Input: part model. Units: mm. Frame: model coordinates. A direction names the side the tool comes from. Coordinates: 2 decimals unless noted, no trailing zeros. Order: outer loops, then holes, each group sorted by start corner. A loop starts at its lowest first (then second) coordinate and runs counter-clockwise, first axis right, second up. Notation, with made-up numbers: M 23,44 L 80,44 A13 cw 80,55 Z; hole C -12.5,10.5 d5. An arc over 180 degrees is marked long. Answer in a Markdown table with one row per item.
from build123d import *

# Parameters (mm, degrees)
SKETCH1_W           = 100
SKETCH1_H           = 100
SKETCH1_R           = 3.5
BOSS_EXTRUDE1_DEPTH = 5
CUT_EXTRUDE1_START  = -5
SKETCH6_R           = 5
CUT_EXTRUDE1_DEPTH  = 3
BOSS_EXTRUDE2_START = 40
SKETCH8_W           = 8
SKETCH8_H           = 58
BOSS_EXTRUDE2_DEPTH = 180
SKETCH9_W           = 180
SKETCH9_H           = 9
BOSS_EXTRUDE3_DEPTH = 230
SKETCH13_R          = 3.5
CUT_EXTRUDE3_DEPTH  = 9
SKETCH15_W          = 6
SKETCH15_H          = 100
BOSS_EXTRUDE6_DEPTH = 73
CUT_EXTRUDE4_REACH  = 309.259
SKETCH16_W          = 130
SKETCH16_H          = 25
FILLET1_R           = 40
FILLET2_R           = 10
SKETCH17_W          = 6
SKETCH17_H          = 20
BOSS_EXTRUDE7_DEPTH = 50
FILLET3_R           = 10
FILLET4_R           = 10
FILLET6_R           = 30
FILLET7_R           = 10
SKETCH18_W          = 10
SKETCH18_H          = 238
BOSS_EXTRUDE8_DEPTH = 20
FILLET8_R           = 10
FILLET9_R           = 10
FILLET10_R          = 5


# Some blends are built 0.0001 mm under size
with BuildPart() as part:
    # Sketch1 → Boss-Extrude1 (new body)
    with BuildSketch(Plane(origin=(0, 0, 0), x_dir=(1, 0, 0), z_dir=(0, 1, 0))):
        Rectangle(SKETCH1_W, SKETCH1_H)
        with Locations(Location((-37.5, 37.5, 0), (0, 0, 270))):
            Circle(SKETCH1_R, mode=Mode.SUBTRACT)
        with Locations(Location((37.5, 37.5, 0), (0, 0, 90))):
            Circle(SKETCH1_R, mode=Mode.SUBTRACT)
        with Locations(Location((37.5, -37.5, 0), (0, 0, 270))):
            Circle(SKETCH1_R, mode=Mode.SUBTRACT)
        with Locations(Location((-37.5, -37.5, 0), (0, 0, 90))):
            Circle(SKETCH1_R, mode=Mode.SUBTRACT)
    extrude(amount=BOSS_EXTRUDE1_DEPTH)

    # Sketch6 → Cut-Extrude1 (cut)
    with BuildSketch(Plane.XZ.offset(CUT_EXTRUDE1_START)):
        with Locations(Location((-37.5, 37.5, 0), (0, 0, 90))):
            Circle(SKETCH6_R)
        with Locations(Location((37.5, 37.5, 0), (0, 0, 90))):
            Circle(SKETCH6_R)
        with Locations(Location((37.5, -37.5, 0), (0, 0, 90))):
            Circle(SKETCH6_R)
        with Locations(Location((-37.5, -37.5, 0), (0, 0, 90))):
            Circle(SKETCH6_R)
    extrude(amount=CUT_EXTRUDE1_DEPTH, mode=Mode.SUBTRACT)

    # Sketch8 → Boss-Extrude2 (add)
    with BuildSketch(Plane.ZY.offset(50).offset(BOSS_EXTRUDE2_START)):
        with Locations((54, 29)):
            Rectangle(SKETCH8_W, SKETCH8_H)
    extrude(amount=-BOSS_EXTRUDE2_DEPTH)

    # Sketch9 → Boss-Extrude3 (add)
    with BuildSketch(Plane.XY.offset(58)):
        with Locations((0, 53.5)):
            Rectangle(SKETCH9_W, SKETCH9_H)
    extrude(amount=BOSS_EXTRUDE3_DEPTH)

    # Sketch13 → Cut-Extrude3 (cut)
    with BuildSketch(Plane(origin=(0, 58, 0), x_dir=(1, 0, 0), z_dir=(0, 1, 0))):
        with Locations(Location((-37.5, -190.5, 0), (0, 0, 270))):
            Circle(SKETCH13_R)
        with Locations(Location((37.5, -190.5, 0), (0, 0, 270))):
            Circle(SKETCH13_R)
        with Locations(Location((37.5, -265.5, 0), (0, 0, 270))):
            Circle(SKETCH13_R)
        with Locations(Location((-37.5, -265.5, 0), (0, 0, 270))):
            Circle(SKETCH13_R)
    extrude(amount=-CUT_EXTRUDE3_DEPTH, mode=Mode.SUBTRACT)

    # Sketch15 → Boss-Extrude6 (add)
    with BuildSketch(Plane(origin=(0, 5, 0), x_dir=(1, 0, 0), z_dir=(0, 1, 0))):
        with Locations((-47, 0)):
            Rectangle(SKETCH15_W, SKETCH15_H)
        with Locations((47, 0)):
            Rectangle(SKETCH15_W, SKETCH15_H)
    extrude(amount=BOSS_EXTRUDE6_DEPTH)

    # Sketch16 → Cut-Extrude4 (cut, up to next)
    with BuildSketch(Plane(origin=(0, 58, 0), x_dir=(1, 0, 0), z_dir=(0, 1, 0)), mode=Mode.PRIVATE) as cut_extrude4_sk1:
        with Locations((0, -130.5)):
            Rectangle(SKETCH16_W, SKETCH16_H)
    cut_extrude4_tool1 = extrude(cut_extrude4_sk1.sketch, amount=-CUT_EXTRUDE4_REACH, mode=Mode.PRIVATE) & part.part
    add(cut_extrude4_tool1.solids().sort_by_distance((0, 58, 130.5))[0], mode=Mode.SUBTRACT)

    # Fillet1
    fillet1_edges = [part.edges().sort_by_distance(p)[0] for p in [
        (0, 49, 58),
    ]]
    fillet(fillet1_edges, radius=FILLET1_R)

    # Fillet2
    fillet2_edges = [part.edges().sort_by_distance(p)[0] for p in [
        (65, 53.5, 118),
        (65, 53.5, 143),
        (-65, 53.5, 143),
        (-65, 53.5, 118),
    ]]
    fillet(fillet2_edges, radius=FILLET2_R)

    # Sketch17 → Boss-Extrude7 (add)
    with BuildSketch(Plane.XY.offset(50)):
        with Locations((-47, 68)):
            Rectangle(SKETCH17_W, SKETCH17_H)
        with Locations((47, 68)):
            Rectangle(SKETCH17_W, SKETCH17_H)
    extrude(amount=BOSS_EXTRUDE7_DEPTH)

    # Fillet3
    fillet3_edges = [part.edges().sort_by_distance(p)[0] for p in [
        (47, 78, 100),
        (-47, 78, 100),
    ]]
    fillet(fillet3_edges, radius=FILLET3_R)

    # Fillet4
    fillet4_edges = [part.edges().sort_by_distance(p)[0] for p in [
        (47, 58, 100),
        (-47, 58, 100),
    ]]
    fillet(fillet4_edges, radius=FILLET4_R - 0.0001)  # a hair under: the kernel refuses the full size

    # Fillet6
    fillet6_edges = [part.edges().sort_by_distance(p)[0] for p in [
        (50, 29, 50),
        (-50, 29, 50),
    ]]
    fillet(fillet6_edges, radius=FILLET6_R)

    # Fillet7
    # the kernel refuses this fillet: 10 mm, written as the material it takes off along each edge
    with BuildSketch(Plane(origin=(-114.974997499, 0, 58), x_dir=(0, 0.9999996667390088, 0.0008164079075175184), z_dir=(1, 0, 0))) as fillet7_piece_1:
        with BuildLine():
            CenterArc((9.991840753, -9.99815975), FILLET7_R, 91.099215266, 88.854008002)
            Line((-0.008155914, -9.989995671), (-1.008155581, -9.989179263))
            Line((-1.008155581, -9.989179263), (-0.999999667, 0.000816408))
            Line((-0.999999667, 0.000816408), (0.000816408, 0.999999667))
            ThreePointArc((0.000816408, 0.999999667), (9.000813409, 0.992651996), (9.780819517, 0.999815975))
            Line((9.780819517, 0.999815975), (9.800003266, 0))
        make_face()
    extrude(amount=229.949994999, mode=Mode.SUBTRACT)

    # Sketch18 → Boss-Extrude8 (add)
    with BuildSketch(Plane(origin=(0, 58, 0), x_dir=(1, 0, 0), z_dir=(0, 1, 0))):
        with Locations((-85, -169)):
            Rectangle(SKETCH18_W, SKETCH18_H)
        with Locations((85, -169)):
            Rectangle(SKETCH18_W, SKETCH18_H)
    extrude(amount=BOSS_EXTRUDE8_DEPTH)

    # Fillet8
    # the kernel refuses this fillet: 10 mm, written as the material it adds along each edge
    with BuildSketch(Plane(origin=(80, 58, 25), x_dir=(0, 1, 0), z_dir=(0, 0, 1))) as fillet8_piece_1_section:
        with BuildLine():
            CenterArc((FILLET8_R, FILLET8_R), FILLET8_R, 180, 90)
            Line((0, FILLET8_R), (0, 0))
            Line((0, 0), (FILLET8_R, 0))
        make_face()
    fillet8_piece_1 = extrude(amount=263, mode=Mode.PRIVATE)
    fillet8_piece_1 = fillet8_piece_1 - Plane(origin=(80, 58.60546515, 20), x_dir=(-1, 0, 0), z_dir=(0, -1, 0)) * Cylinder(30, 567, mode=Mode.PRIVATE)
    add(fillet8_piece_1)
    with BuildSketch(Plane(origin=(-80, 58, 25), x_dir=(0, 1, 0), z_dir=(0, 0, 1))) as fillet8_piece_2_section:
        with BuildLine():
            CenterArc((FILLET8_R, -FILLET8_R), FILLET8_R, 90, 90)
            Line((0, -FILLET8_R), (0, 0))
            Line((0, 0), (FILLET8_R, 0))
        make_face()
    fillet8_piece_2 = extrude(amount=263, mode=Mode.PRIVATE)
    fillet8_piece_2 = fillet8_piece_2 - Plane(origin=(-80, 58.605465201, 20), x_dir=(0, 0, 1), z_dir=(0, -1, 0)) * Cylinder(30, 567, mode=Mode.PRIVATE)
    add(fillet8_piece_2)
    # the kernel refuses this fillet: 10 mm, written as the material it takes off along each edge
    with BuildSketch(Plane(origin=(90, 49, 98), x_dir=(-1, 0, 0), z_dir=(0, 0, 1))) as fillet8_2_piece_1:
        with BuildLine():
            CenterArc((FILLET8_R, -FILLET8_R), FILLET8_R, 90, 90)
            Line((0, -FILLET8_R), (0, 0))
            Line((0, 0), (FILLET8_R, 0))
        make_face()
    extrude(amount=215, mode=Mode.SUBTRACT)
    with BuildSketch(Plane(origin=(90, 10, 48.010001), x_dir=(0, 0.6665779251845226, -0.7454353557866013), z_dir=(0, 0.7454353557866013, 0.6665779251845226))) as fillet8_2_piece_2:
        with BuildLine():
            CenterArc((10 - FILLET8_R, FILLET8_R), FILLET8_R, 270, 90)
            Line((10 - FILLET8_R, 0), (10, 0))
            Line((10, 0), (10, FILLET8_R))
        make_face()
    revolve(axis=Axis((90, 10, 48.010001), (-1, 0, 0)), revolution_arc=220.657501671, mode=Mode.SUBTRACT)
    with BuildSketch(Plane(origin=(-90, 10, 48.010001), x_dir=(0, 0.6665779251845226, -0.7454353557866013), z_dir=(0, 0.7454353557866013, 0.6665779251845226))) as fillet8_2_piece_3:
        with BuildLine():
            CenterArc((10 - FILLET8_R, -FILLET8_R), FILLET8_R, 0, 90)
            Line((10 - FILLET8_R, 0), (10, 0))
            Line((10, 0), (10, -FILLET8_R))
        make_face()
    revolve(axis=Axis((-90, 10, 48.010001), (-1, 0, 0)), revolution_arc=220.657501671, mode=Mode.SUBTRACT)
    with BuildSketch(Plane(origin=(-90, 49, 98), x_dir=(1, 0, 0), z_dir=(0, 0, 1))) as fillet8_2_piece_4:
        with BuildLine():
            CenterArc((FILLET8_R, FILLET8_R), FILLET8_R, 180, 90)
            Line((0, FILLET8_R), (0, 0))
            Line((0, 0), (FILLET8_R, 0))
        make_face()
    extrude(amount=215, mode=Mode.SUBTRACT)
    with BuildSketch(Plane(origin=(90, 9, 98), x_dir=(0, 0.019999999999999886, -0.999799979995999), z_dir=(0, -0.999799979995999, -0.019999999999999886))) as fillet8_2_piece_5:
        with BuildLine():
            CenterArc((40 + FILLET8_R, -FILLET8_R), FILLET8_R, 90, 90)
            Line((40 + FILLET8_R, 0), (40, 0))
            Line((40, 0), (40, -FILLET8_R))
        make_face()
    revolve(axis=Axis((90, 9, 98), (1, 0, 0)), revolution_arc=88.854008002, mode=Mode.SUBTRACT)
    with BuildSketch(Plane(origin=(-90, 9, 98), x_dir=(0, 0.019999999999999886, -0.999799979995999), z_dir=(0, -0.999799979995999, -0.019999999999999886))) as fillet8_2_piece_6:
        with BuildLine():
            CenterArc((40 + FILLET8_R, FILLET8_R), FILLET8_R, 180, 90)
            Line((40 + FILLET8_R, 0), (40, 0))
            Line((40, 0), (40, FILLET8_R))
        make_face()
    revolve(axis=Axis((-90, 9, 98), (1, 0, 0)), revolution_arc=88.854008002, mode=Mode.SUBTRACT)

    # Fillet9
    fillet9_edges = [part.edges().sort_by_distance(p)[0] for p in [
        (50, 58, 64.99995),
        (-50, 58, 64.99995),
    ]]
    fillet(fillet9_edges, radius=FILLET9_R)

    # Fillet10
    fillet10_edges = [part.edges().sort_by_distance(p)[0] for p in [
        (-90, 78, 169),
        (-85, 78, 288),
        (-80, 78, 169),
        (-85, 78, 50),
        (90, 78, 169),
        (85, 78, 50),
        (80, 78, 169),
        (85, 78, 288),
    ]]
    fillet(fillet10_edges, radius=FILLET10_R - 0.0001)  # a hair under: the kernel refuses the full size


solid = part.part
1) Reachability of faces 4 (the face through (-77.15, 61.01, 166.46)), 5 (the face through (62.15, 53.44, 121.01)), 6 (the face through (-44, 41, 11)), 7 (the face through (-1, 49, 192)), 8 (the face through (37.28, 3.521, -42.495)) from +Z, -Z, +X, -X, +Y, -Y: full face, straight path, thin tool, end or side. Return the list, or none.
Resolved:
| item | result |
|---|---|
| face 4 | +Z, -Z, +Y |
| face 5 | +Y, -Y |
| face 6 | -Z, +Y |
| face 7 | +Z, +X, -X, -Y |
| face 8 | +Y |
2) Cut plane D-D, the plane z = 37.5. Output: boundary loops of the cut face in (x, y).
Resolved:
| item | result |
|---|---|
| outline | M -55.63,0 L -41,0 L -41,2 L -42.5,2 L -42.5,5 L -44,5 L -44,78 L -50,78 L -50,68 A10 cw -55.63,59 Z; M -34,0 L 34,0 L 34,2 L 32.5,2 L 32.5,5 L -32.5,5 L -32.5,2 L -34,2 Z; M 41,0 L 55.63,0 L 55.63,59 A10 cw 50,68 L 50,78 L 44,78 L 44,5 L 42.5,5 L 42.5,2 L 41,2 Z |
3) Contact query for flat-ended pins moving along their axis: pin 1 (8 mm diameter, centred on x = 38, z = -35.5, fed in from +Y); pin 2 (1 mm diameter, centred on x = -50, z = 108.5, fed in from -Y); pin 3 (3 mm diameter, centred on y = 51.5, z = 151, fed in from -X); pin 4 (4 mm diameter, centred on x = 65, y = 61, fed in from -Z). Output: stop coordinate, or through.
Resolved:
| item | result |
|---|---|
| pin 1 | stops at y = 5 |
| pin 2 | stops at y = 49 |
| pin 3 | stops at x = -88 |
| pin 4 | passes through |
4) Mould query, pull axis X, two halves, no side actions, for faces 1 (the face through (86.99, 51.85, 191.67)), 2 (the face through (-8, 4, -50)), 3 (the face through (-62.15, 53.44, 139.99)). Classes: +X half, -X half, draft (parallel to the pull), parting line (faces both ways), or undercut.
Resolved:
| item | result |
|---|---|
| face 1 | +X half |
| face 2 | draft |
| face 3 | undercut |
5) Cut plane A-A, the plane z = 265.5. State how many separate pieces and enclosed holes the cut face has, and give its area (3 significant figures).
Resolved:
| item | result |
|---|---|
| separate pieces | 3 |
| enclosed holes | 0 |
| area | 1,870 mm2 |
6) Cut plane C-C, the plane z = -22. Output: boundary loops of the cut face in (x, y).
Resolved:
| item | result |
|---|---|
| outline | M -50,0 L 50,0 L 50,78 L 44,78 L 44,5 L -44,5 L -44,78 L -50,78 Z |
7) Material intervals for probe 1 along Z at (x, y) = (37, 52); probe 2 along X at (y, z) = (4.15, -37.5); probe 3 along X at (y, z) = (54, 190.5), sorted ascending.
Resolved:
| item | result |
|---|---|
| probe 1 | z = 50 to 118, 143 to 187.04, 193.96 to 262.04, 268.96 to 288 |
| probe 2 | x = -50 to -42.5, -32.5 to 32.5, 42.5 to 50 |
| probe 3 | x = -88.66 to -41, -34 to 34, 41 to 88.66 |
